Check sheet for the modelled part. Datum: model origin and axes. Units: mm. A direction names the side the tool comes from. Round coordinates to 2 decimals unless told otherwise and drop trailing zeros. Loops run counter-clockwise (first coordinate to the right, second up) from the corner with the lowest first, then second, coordinate; pieces in that order, holes last. Notation, with made-up numbers: (41.5, 56.25) - (52.5, 56.25) arc R22 ccw to (52.5, 88.25) - close; hole circle Ø11 at (17, 46.5). An arc over 180 degrees is marked (long way). Return JSON: item names as keys, results as strings.
from build123d import *

# Parameters (mm, degrees)
F2_R     = 4.7625
F3_DEPTH = 19.05


with BuildPart() as f3:
    # F2 (on Right) → F3 (new body)
    with BuildSketch(Plane.YZ):
        with BuildLine():
            ThreePointArc((-1024.607466, 699.474183), (-1058.459537, 691.137771), (-1052.101189, 656.859061))
            Line((-1052.101189, 656.859061), (-841.879547, 503.255308))
            Line((-841.879547, 503.255308), (-735.705726, 280.30051))
            ThreePointArc((-735.705726, 280.30051), (-702.74925, 267.882869), (-689.064049, 300.333483))
            Line((-689.064049, 300.333483), (-700.258076, 329.45928))
            Line((-700.258076, 329.45928), (-693.145152, 340.503097))
            Line((-693.145152, 340.503097), (-714.197453, 407.111138))
            Line((-714.197453, 407.111138), (-714.197453, 438.202467))
            Line((-714.197453, 438.202467), (-734.424889, 453.702241))
            Line((-734.424889, 453.702241), (-795.707226, 569.954991))
            Line((-795.707226, 569.954991), (-1024.607466, 699.474183))
        make_face()
        with Locations((-712.773263, 291.221231)):
            Circle(F2_R, mode=Mode.SUBTRACT)
        with Locations((-723.694212, 436.423379)):
            Circle(F2_R, mode=Mode.SUBTRACT)
        with Locations((-1037.116024, 677.367714)):
            Circle(F2_R, mode=Mode.SUBTRACT)
        with Locations((-1007.925361, 660.266367)):
            Circle(F2_R, mode=Mode.SUBTRACT)
        with Locations((-826.159707, 542.639145)):
            Circle(F2_R, mode=Mode.SUBTRACT)
    extrude(amount=F3_DEPTH)


solid = f3.part
Q1. Sectioned sample at C-C (z = 581). Enter the section's corners in (x, y), plus the area to 3 significant figures.
Answer key:
{"outline": "(0, -948.28) - (19.05, -948.28) - (19.05, -815.23) - (0, -815.23) - close", "area": "2,530 mm²"}
Q2. Depth check by flat-ended pin: P1, Ø1.5, axis at x = 13.5, y = -904, coming from the -Z side; P2, Ø2, axis at x = 8.5, y = -856.5, coming from the -Z side; P3, Ø2, axis at x = 5, y = -920.5, coming from the +Z side. Enter the tip coordinate at first touch or a pass-through.
Answer key:
{"P1": "stops at z = 548.1", "P2": "stops at z = 513.21", "P3": "stops at z = 641.13"}
Q3. Scan lines: probe 1 along Z at (x, y) = (3.25, -1010.5); probe 2 along Z at (x, y) = (10.25, -1033); probe 3 along Y at (x, z) = (1.5, 556.5). Record each from-to range of solid material in increasing order. Write a range as [from, to].
Answer key:
{"probe 1": "z = [626.46, 656.26], [664.27, 691.49]", "probe 2": "z = [642.9, 674.97], [679.76, 702.43]", "probe 3": "y = [-914.75, -788.61]"}
Q4. Tool access check on faces 5 (the face through (9.392, -789.536, 393.339)), 6 (the face through (9.39, -694.58, 314.69)). Record the directions out of +Z, -Z, +X, -X, +Y, -Y that give a thin tool (end or side, any length) a straight path to the whole face; none if there is none.
Answer key:
{"face 5": "-Z, +X, -X, -Y", "face 6": "+X, -X, +Y"}
Q5. Sectioned sample at B-B (y = -910). Enter the section's corners in (x, z).
Answer key:
{"outline": "(0, 553.03) - (19.05, 553.03) - (19.05, 634.63) - (0, 634.63) - close"}
Q6. Draft check along Y on faces 1 (the face through (9.392, -823.599, 546.655)), 2 (the face through (9.39, -948.46, 581.13)), 3 (the face through (9.392, -1011.705, 657.368)), 4 (the face through (9, -714.197, 422)). Enter one of: released by +Y, released by -Y, zero draft, split by the parting line, or undercut.
Answer key:
{"face 1": "undercut", "face 2": "released by -Y", "face 3": "undercut", "face 4": "released by +Y"}
Q7. Sectioned sample at A-A (x = 14.75). Enter the section's corners in (y, z) (1 decimal).
Answer key:
{"outline": "(-1052.1, 656.9) - (-841.9, 503.3) - (-735.7, 280.3) arc R25.4 ccw to (-689.1, 300.3) - (-700.3, 329.5) - (-693.1, 340.5) - (-714.2, 407.1) - (-714.2, 438.2) - (-734.4, 453.7) - (-795.7, 570) - (-1024.6, 699.5) arc R25.4 ccw to start; hole circle Ø9.5 at (-1037.1, 677.4); hole circle Ø9.5 at (-1007.9, 660.3); hole circle Ø9.5 at (-826.2, 542.6); hole circle Ø9.5 at (-723.7, 436.4); hole circle Ø9.5 at (-712.8, 291.2)"}
